Can you work these out from the model? Positions are in its coordinate system, mm. A direction names the side the tool comes from. Give positions to 0.01 mm unless a question says otherwise; leave off trailing zeros. Loops run counter-clockwise (first coordinate to the right, second up) from the corner with the lowest first, then second, coordinate; pieces in that order, holes last. Notation, with made-up numbers: M 59,30.5 L 64,30.5 A14 ccw 64,36.5 Z; hole C -34,88 d3. An arc over 180 degrees is marked long. Put each result on its own line as item: value. Start each with the question number.
1) For P1, Ø11, axis at x = 15.5, z = 2, coming from the +Y side; P2, Ø6, axis at x = 9, y = -3, coming from the +Z side; P3, Ø4, axis at x = -0.5, z = 8.5, coming from the +Y side, each with a flat end and sliding along its axis, tell me the tip position at first contact or that it passes through.
2) Please list where these lines run through material, in increasing order: line 1 along X through (y, z) = (-2.75, 0); line 2 along X through (y, z) = (-5, -7.5); line 3 along X through (y, z) = (-3.25, 0.5). Write a range as from..to.
3) Imagine slicing it at A-A (y = -4.25). Write out the boundary of the cut face in (x, z).
4) If we mould it in two halves opening along Z, with no side actions, what happens to faces 6 (the cylindrical face through (26.925, -2.382, -0.683)), 7 (the flat face through (0, -5, -10)), 8 (the cylindrical face through (0.421, -4.935, 8.972)), 9 (the flat face through (0, -5, 10))? For each: +Z half, -Z half, draft (parallel to the pull), parting line (faces both ways), or undercut.
5) Imagine slicing it at C-C (z = 0). Write out the boundary of the cut face in (x, y), then the cut area to 3 significant figures.
6) Imagine slicing it at B-B (x = -15). Write out the boundary of the cut face in (y, z), then the cut area to 3 significant figures.
7) For faces 1 (the flat face through (-10, -5, -7)), 2 (the flat face through (20, -0.65, 0)), 3 (the flat face through (30, -3.75, -8)), 4 (the flat face through (-5, 3, 0)), 5 (the flat face through (-15, -3.75, 7)), which set-ups out of +Z, -Z, +X, -X, +Y, -Y let a thin tool reach every point of the face, with its end or its side?
8) Imagine slicing it at D-D (x = 0). Write out the boundary of the cut face in (y, z), then the cut area to 3 significant figures.
from build123d import *
from OCP.BRepFilletAPI import BRepFilletAPI_MakeChamfer

# Parameters (mm, degrees)
SKETCH1_W           = 55
SKETCH1_H           = 20
BOSS_EXTRUDE1_DEPTH = 6.5
SKETCH2_W           = 10
SKETCH2_H           = 10
CUT_EXTRUDE3_DEPTH  = 7.15
SKETCH6_W           = 55
SKETCH6_H           = 5
CUT_EXTRUDE4_DEPTH  = 3.1
SKETCH7_R           = 1.6
CUT_EXTRUDE5_DEPTH  = 10
SKETCH9_W           = 5
SKETCH9_H           = 5
SKETCH9_W_2         = 20
CUT_EXTRUDE6_DEPTH  = 3
SKETCH10_R          = 1.4
CUT_EXTRUDE7_DEPTH  = 3
CHAMFER1_SIZE       = 0.2
CHAMFER1_SIZE2      = 0.346410162
SKETCH12_R          = 3.15
CUT_EXTRUDE8_DEPTH  = 3
CHAMFER2_SIZE       = 0.5
CHAMFER2_SIZE2      = 0.233153829


with BuildPart() as part:
    # Sketch1 → Boss-Extrude1 (new, symmetric)
    with BuildSketch(Plane(origin=(0, 0, 0), x_dir=(1, 0, 0), z_dir=(0, 1, 0))):
        with Locations((7.5, 0)):
            Rectangle(SKETCH1_W, SKETCH1_H)
    extrude(amount=BOSS_EXTRUDE1_DEPTH, both=True)

    # Sketch2 → Cut-Extrude3 (cut)
    with BuildSketch(Plane(origin=(0, 6.5, 0), x_dir=(1, 0, 0), z_dir=(0, 1, 0))):
        Polygon((-5, -10), (-20, -10), (-20, 10), (-5, 10), (5, 10), (35, 10), (35, -10), (5, -10), align=None)
        Rectangle(SKETCH2_W, SKETCH2_H, mode=Mode.SUBTRACT)
    extrude(amount=-CUT_EXTRUDE3_DEPTH, mode=Mode.SUBTRACT)

    # Sketch6 → Cut-Extrude4 (cut)
    with BuildSketch(Plane(origin=(0, -0.65, 0), x_dir=(1, 0, 0), z_dir=(0, 1, 0))):
        with Locations((7.5, -7.5)):
            Rectangle(SKETCH6_W, SKETCH6_H)
        Polygon((-5, 5), (-20, 5), (-20, 10), (35, 10), (35, 5), align=None)
    extrude(amount=-CUT_EXTRUDE4_DEPTH, mode=Mode.SUBTRACT)

    # Sketch7 → Cut-Extrude5 (cut)
    with BuildSketch(Plane.XZ.offset(6.5)):
        with Locations(Location((-15, 0, 0), (0, 0, 270))):
            Circle(SKETCH7_R)
    extrude(amount=-CUT_EXTRUDE5_DEPTH, mode=Mode.SUBTRACT)

    # Sketch9 → Cut-Extrude6 (cut)
    with BuildSketch(Plane(origin=(0, -3.75, 0), x_dir=(1, 0, 0), z_dir=(0, 1, 0))):
        with Locations((-7.5, 7.5)):
            Rectangle(SKETCH9_W, SKETCH9_H)
        with Locations((-7.5, -7.5)):
            Rectangle(SKETCH9_W, SKETCH9_H)
        with Locations((15, 7.5)):
            Rectangle(SKETCH9_W_2, SKETCH9_H)
        with Locations((15, -7.5)):
            Rectangle(SKETCH9_W_2, SKETCH9_H)
    extrude(amount=-CUT_EXTRUDE6_DEPTH, mode=Mode.SUBTRACT)

    # Sketch10 → Cut-Extrude7 (cut)
    with BuildSketch(Plane(origin=(0, -3.75, 0), x_dir=(1, 0, 0), z_dir=(0, 1, 0))):
        with Locations(Location((0, 7.636752006, 0), (0, 0, 270))):
            Circle(SKETCH10_R)
        with Locations(Location((0, -7.636752006, 0), (0, 0, 270))):
            Circle(SKETCH10_R)
    extrude(amount=-CUT_EXTRUDE7_DEPTH, mode=Mode.SUBTRACT)

    # Chamfer1: one chamfer whose edges measure the first distance from different faces: ONE call of the kernel's chamfer builder (chamfer() names one face for all edges)
    chamfer1_edges_1 = [part.edges().sort_by_distance(p)[0] for p in [
        (0, -6.5, 6.236752006),
        (-15, -6.5, 1.6),
    ]]
    chamfer1_side_1 = [part.faces().sort_by_distance(p)[0] for p in [
        (6.925437522, -6.5, 0),
    ]]
    chamfer1_edges_2 = [part.edges().sort_by_distance(p)[0] for p in [
        (0, -6.5, -9.036752006),
    ]]
    chamfer1_side_2 = [part.faces().sort_by_distance(p)[0] for p in [
        (0, -5.125, -9.036752006),
    ]]
    chamfer1_edges_3 = [part.edges().sort_by_distance(p)[0] for p in [
        (-15, -0.65, 1.6),
    ]]
    chamfer1_side_3 = [part.faces().sort_by_distance(p)[0] for p in [
        (-12.358364724, -0.65, 0),
    ]]
    chamfer1 = BRepFilletAPI_MakeChamfer(part.part.solid().wrapped)
    for e in chamfer1_edges_1:
        chamfer1.Add(CHAMFER1_SIZE, CHAMFER1_SIZE2, e.wrapped, chamfer1_side_1[0].wrapped)  # the first distance lies on this face
    for e in chamfer1_edges_2:
        chamfer1.Add(CHAMFER1_SIZE, CHAMFER1_SIZE2, e.wrapped, chamfer1_side_2[0].wrapped)  # the first distance lies on this face
    for e in chamfer1_edges_3:
        chamfer1.Add(CHAMFER1_SIZE, CHAMFER1_SIZE2, e.wrapped, chamfer1_side_3[0].wrapped)  # the first distance lies on this face
    add(Compound.cast(chamfer1.Shape()), mode=Mode.REPLACE)

    # Sketch12 → Cut-Extrude8 (cut)
    with BuildSketch(Plane(origin=(0, -0.65, 0), x_dir=(1, 0, 0), z_dir=(0, 1, 0))):
        with Locations(Location((30, 0, 0), (0, 0, 270))):
            Circle(SKETCH12_R)
    extrude(amount=-CUT_EXTRUDE8_DEPTH, mode=Mode.SUBTRACT)

    # Chamfer2
    chamfer2_edges = [part.edges().sort_by_distance(p)[0] for p in [
        (30, -0.65, -3.15),
    ]]
    chamfer2_side = [part.faces().sort_by_distance(p)[0] for p in [
        (30, -2.15, -3.15),
    ]]
    chamfer(chamfer2_edges, length=CHAMFER2_SIZE, length2=CHAMFER2_SIZE2, reference=chamfer2_side[0])


solid = part.part
Recorded:
1. P1: y = -0.65
1. P2: z = 5
1. P3: y = -3.75
2. line 1: -20..-16.6, -13.4..26.85, 33.15..35
2. line 2: -20..-10, -5..-1.39, 1.39..5, 25..35
2. line 3: -20..-16.52, -13.48..26.89, 33.11..35
3. outline: M -20,-10 L -10,-10 L -10,-5 L -5,-5 L -5,-10 L 5,-10 L 5,-5 L 25,-5 L 25,-10 L 35,-10 L 35,10 L 25,10 L 25,5 L 5,5 L 5,10 L -5,10 L -5,5 L -10,5 L -10,10 L -20,10 Z; hole C -15,0 d3.2; hole C 0,-7.64 d2.8; hole C 0,7.64 d2.8
4. face 6: undercut
4. face 7: -Z half
4. face 8: undercut
4. face 9: +Z half
5. outline: M -20,-6.5 L -16.8,-6.5 L -16.6,-6.15 L -16.6,-1 L -16.8,-0.65 L -20,-0.65 Z; M -13.4,-6.15 L -13.2,-6.5 L 35,-6.5 L 35,-0.65 L 33.38,-0.65 L 33.15,-1.15 L 33.15,-3.65 L 26.85,-3.65 L 26.85,-1.15 L 26.62,-0.65 L 5,-0.65 L 5,6.5 L -5,6.5 L -5,-0.65 L -13.2,-0.65 L -13.4,-1 Z
5. area: 355 mm²
6. outline: M -6.5,-10 L -3.75,-10 L -3.75,-5 L -0.65,-5 L -0.65,-1.8 L -1,-1.6 L -6.15,-1.6 L -6.5,-1.8 Z; M -6.5,1.8 L -6.15,1.6 L -1,1.6 L -0.65,1.8 L -0.65,5 L -3.75,5 L -3.75,10 L -6.5,10 Z
6. area: 67.1 mm²
7. face 1: -Z, +Y, -Y
7. face 2: +Z, -Z, +X, +Y
7. face 3: -Z, +X, -X, +Y
7. face 4: +Z, -Z, -X, +Y
7. face 5: +Z, +X, -X, +Y
8. outline: M -6.5,-10 L -3.75,-10 L -3.75,-9.04 L -6.3,-9.04 L -6.5,-9.38 Z; M -6.5,-5.89 L -6.3,-6.24 L -3.75,-6.24 L -3.75,-5 L 6.5,-5 L 6.5,5 L -3.75,5 L -3.75,6.24 L -6.15,6.24 L -6.5,6.04 Z; M -6.5,9.24 L -6.15,9.04 L -3.75,9.04 L -3.75,10 L -6.5,10 Z
8. area: 142 mm²
